Read the model definition and answer for the solid it produces. Units are mm, in the model's axes. A direction names the side the tool comes from. Round coordinates to 2 decimals unless told otherwise and drop trailing zeros. Order: outer loops, then holes, each group sorted by start corner. A loop starts at its lowest first (then second) coordinate and runs counter-clockwise, first axis right, second up. Notation, with made-up numbers: (61, 0.25) -> (66, 0.25) arc R15 ccw to (66, 17.25) -> close; hole circle Ø11 at (20.5, 50). An arc over 180 degrees is marked (long way). Answer as a JSON object with one key per item and string values. Group by question number.
Item 1: Section C-C, the plane y = 12.5 is taken. Write down the section's boundary in (x, z).
Item 2: For faces 1 (the cylindrical face through (8.26, 3.83, -4.3)), 2 (the cylindrical face through (9.476, 3.368, 10.331)), 3 (the flat face through (67, 0, -14)), 4 (the flat face through (-1, 16, 0)), determine the directions among +Z, -Z, +X, -X, +Y, -Y from which every point of the face is accessible in a straight line to the end or side of a thin tool.
Item 3: Consider probe 1 along Z at (x, y) = (11, -1.5); probe 2 along Z at (x, y) = (37, -10); probe 3 along X at (y, z) = (-6, 1). Determine where each line is inside the solid, lowest interval first. Write a range as from..to.
Item 4: Section A-A, the plane z = -10 is taken. Write down the section's boundary in (x, y), plus the area to 3 significant figures.
Item 5: Section B-B, the plane x = 37 is taken. Write down the section's boundary in (y, z).
Item 6: The mould has two halves that part along Z. Classify faces 5 (the flat face through (-1, -16, 0)), 6 (the flat face through (93, 0, -16)), 7 (the cylindrical face through (-62, 4, -5)): pulls with the +Z half, pulls with the -Z half, needs draft (parallel to the pull), parting line crosses it, or undercut.
Item 7: Given P1, Ø3, axis at x = 11, y = 4, coming from the +Z side; P2, Ø2, axis at x = -87, z = 0, coming from the +Y side; P3, Ø6, axis at x = -63, z = 0, coming from the +Y side, each flat-ended and moving along its own axis, determine where each tip first touches the part or whether it passes through.
from build123d import *

# Parameters (mm, degrees)
SKETCH1_W                                            = 190
SKETCH1_H                                            = 32
BOSS_EXTRUDE1_DEPTH                                  = 16
SKETCH2_W                                            = 25
SKETCH2_H                                            = 4
CUT_EXTRUDE1_DEPTH                                   = 102.513545894
M12_TAPPED_HOLE1_D                                   = 10.2
M12_TAPPED_HOLE1_DEPTH                               = 24
M12_TAPPED_HOLE1_TIP                                 = 3.064389157
M4_TAPPED_HOLE1_D                                    = 3.3
M4_TAPPED_HOLE1_DEPTH                                = 11.5
M4_TAPPED_HOLE1_TIP                                  = 0.991420021
SKETCH13_R                                           = 3
CUT_EXTRUDE2_DEPTH                                   = 102.51354591
CSK_FOR_M4_COUNTERSUNK_FLAT_HEAD_SCREW1_D            = 1.5
CSK_FOR_M4_COUNTERSUNK_FLAT_HEAD_SCREW1_DEPTH        = 10
CSK_FOR_M4_COUNTERSUNK_FLAT_HEAD_SCREW1_CSINK_D      = 4
CSK_FOR_M4_COUNTERSUNK_FLAT_HEAD_SCREW1_CSINK_ANGLE  = 90
CSK_FOR_M4_COUNTERSUNK_FLAT_HEAD_SCREW1_TIP          = 0.450645464
M4_TAPPED_HOLE3_D                                    = 3.3
M4_TAPPED_HOLE3_DEPTH                                = 16
M4_TAPPED_HOLE3_CSINK_D                              = 4
M4_TAPPED_HOLE3_CSINK_ANGLE                          = 90
M4_TAPPED_HOLE3_TIP                                  = 0.991420021
SKETCH26_R                                           = 3
CUT_EXTRUDE4_DEPTH                                   = 32
CSK_FOR_M10_COUNTERSUNK_FLAT_HEAD_SCREW3_D           = 6.5
CSK_FOR_M10_COUNTERSUNK_FLAT_HEAD_SCREW3_CSINK_D     = 13
CSK_FOR_M10_COUNTERSUNK_FLAT_HEAD_SCREW3_CSINK_ANGLE = 90
CHAMFER3_SIZE                                        = 2


with BuildPart() as part:
    # Sketch1 → Boss-Extrude1 (new, symmetric)
    with BuildSketch(Plane.XY):
        Rectangle(SKETCH1_W, SKETCH1_H)
    extrude(amount=BOSS_EXTRUDE1_DEPTH, both=True)

    # Sketch2 → Cut-Extrude1 (cut, through all)
    with BuildSketch(Plane(origin=(0, 16, 0), x_dir=(1, 0, 0), z_dir=(0, 1, 0))):
        with Locations((79.5, 14)):
            Rectangle(SKETCH2_W, SKETCH2_H)
    extrude(amount=-CUT_EXTRUDE1_DEPTH, mode=Mode.SUBTRACT)

    # M12 Tapped Hole1
    with Locations(Plane(origin=(0, 16, 0), x_dir=(1, 0, 0), z_dir=(0, 1, 0))):
        with Locations((-63, 0), (11, 0)):
            Hole(M12_TAPPED_HOLE1_D / 2, depth=M12_TAPPED_HOLE1_DEPTH)
            with Locations((0, 0, -(M12_TAPPED_HOLE1_DEPTH + M12_TAPPED_HOLE1_TIP / 2))):  # 118° drill point
                Cone(0, M12_TAPPED_HOLE1_D / 2, M12_TAPPED_HOLE1_TIP, mode=Mode.SUBTRACT)

    # M4 Tapped Hole1
    with Locations(Plane.XY.offset(16)):
        with Locations((-63, 4), (11, 4)):
            Hole(M4_TAPPED_HOLE1_D / 2, depth=M4_TAPPED_HOLE1_DEPTH)
            with Locations((0, 0, -(M4_TAPPED_HOLE1_DEPTH + M4_TAPPED_HOLE1_TIP / 2))):  # 118° drill point
                Cone(0, M4_TAPPED_HOLE1_D / 2, M4_TAPPED_HOLE1_TIP, mode=Mode.SUBTRACT)

    # Sketch13 → Cut-Extrude2 (cut, through all)
    with BuildSketch(Plane.XY.offset(16)):
        with Locations((-87, 6)):
            Circle(SKETCH13_R)
    extrude(amount=-CUT_EXTRUDE2_DEPTH, mode=Mode.SUBTRACT)

    # CSK for M4 Countersunk Flat Head Screw1
    with Locations(Plane(origin=(0, 16, 0), x_dir=(1, 0, 0), z_dir=(0, 1, 0))):
        with Locations((-87, 0)):
            CounterSinkHole(CSK_FOR_M4_COUNTERSUNK_FLAT_HEAD_SCREW1_D / 2, CSK_FOR_M4_COUNTERSUNK_FLAT_HEAD_SCREW1_CSINK_D / 2, depth=CSK_FOR_M4_COUNTERSUNK_FLAT_HEAD_SCREW1_DEPTH, counter_sink_angle=CSK_FOR_M4_COUNTERSUNK_FLAT_HEAD_SCREW1_CSINK_ANGLE)
            with Locations((0, 0, -(CSK_FOR_M4_COUNTERSUNK_FLAT_HEAD_SCREW1_DEPTH + CSK_FOR_M4_COUNTERSUNK_FLAT_HEAD_SCREW1_TIP / 2))):  # 118° drill point
                Cone(0, CSK_FOR_M4_COUNTERSUNK_FLAT_HEAD_SCREW1_D / 2, CSK_FOR_M4_COUNTERSUNK_FLAT_HEAD_SCREW1_TIP, mode=Mode.SUBTRACT)

    # M4 Tapped Hole3
    with Locations(Plane(origin=(0, 16, 0), x_dir=(1, 0, 0), z_dir=(0, 1, 0))):
        with Locations((-43, 0)):
            CounterSinkHole(M4_TAPPED_HOLE3_D / 2, M4_TAPPED_HOLE3_CSINK_D / 2, depth=M4_TAPPED_HOLE3_DEPTH, counter_sink_angle=M4_TAPPED_HOLE3_CSINK_ANGLE)
            with Locations((0, 0, -(M4_TAPPED_HOLE3_DEPTH + M4_TAPPED_HOLE3_TIP / 2))):  # 118° drill point
                Cone(0, M4_TAPPED_HOLE3_D / 2, M4_TAPPED_HOLE3_TIP, mode=Mode.SUBTRACT)

    # Sketch26 → Cut-Extrude4 (cut)
    with BuildSketch(Plane(origin=(0, 16, 0), x_dir=(1, 0, 0), z_dir=(0, 1, 0))):
        with Locations(Location((-37, 10, 0), (0, 0, 180))):
            Circle(SKETCH26_R)
        with Locations(Location((37, 10, 0), (0, 0, 180))):
            Circle(SKETCH26_R)
    extrude(amount=-CUT_EXTRUDE4_DEPTH, mode=Mode.SUBTRACT)

    # CSK for M10 Countersunk Flat Head Screw3 (through all)
    with Locations(Plane.XY.offset(16)):
        with Locations((79.5, 4)):
            CounterSinkHole(CSK_FOR_M10_COUNTERSUNK_FLAT_HEAD_SCREW3_D / 2, CSK_FOR_M10_COUNTERSUNK_FLAT_HEAD_SCREW3_CSINK_D / 2, counter_sink_angle=CSK_FOR_M10_COUNTERSUNK_FLAT_HEAD_SCREW3_CSINK_ANGLE)

    # Chamfer3
    chamfer3_edges = [part.edges().sort_by_distance(p)[0] for p in [
        (95, 0, 16),
        (-95, 0, 16),
        (-95, 0, -16),
    ]]
    chamfer(chamfer3_edges, length=CHAMFER3_SIZE)


solid = part.part
Values found:
{
 "1": {"outline": "(-95, -14) -> (-93, -16) -> (67, -16) -> (67, -12) -> (92, -12) -> (92, -16) -> (95, -16) -> (95, 14) -> (93, 16) -> (-93, 16) -> (-95, 14) -> close; hole circle Ø1.5 at (-87, 0); hole circle Ø10.2 at (-63, 0); hole circle Ø3.3 at (-43, 0); hole circle Ø6 at (-37, -10); hole circle Ø10.2 at (11, 0); hole circle Ø6 at (37, -10)"},
 "2": {"face 1": "+Y", "face 2": "+Z", "face 3": "-Z, +Y, -Y", "face 4": "+Z, -Z, +X, -X, +Y"},
 "3": {"probe 1": "-16..-5.1, 5.1..16", "probe 2": "-16..-13, -7..16", "probe 3": "-95..-68, -58..6, 16..95"},
 "4": {"outline": "(-95, -16) -> (-40, -16) -> (-40, 16) -> (-95, 16) -> close; (-34, -16) -> (34, -16) -> (34, 16) -> (-34, 16) -> close; (40, -16) -> (95, -16) -> (95, 16) -> (40, 16) -> close; hole circle Ø6 at (-87, 6); hole circle Ø6.5 at (79.5, 4)", "area": "5,630 mm2"},
 "5": {"outline": "(-16, -16) -> (16, -16) -> (16, -13) -> (-16, -13) -> close; (-16, -7) -> (16, -7) -> (16, 16) -> (-16, 16) -> close"},
 "6": {"face 5": "needs draft", "face 6": "pulls with the -Z half", "face 7": "undercut"},
 "7": {"P1": "z = -4.87", "P2": "y = 15", "P3": "y = -9.26"}
}
